Verification items for the finished model (mm, model axes). Face numbers are marked on the shaded views. Round coordinates to 2 decimals unless told otherwise and drop trailing zeros. Write each loop counter-clockwise with the first axis right and the second up, starting at its lowest first coordinate (ties: lowest second). Pieces come first, ordered by that corner, then holes. Notation, with made-up numbers: M 33,35.5 L 86,35.5 A14 ccw 86,60.5 Z; hole C 47.5,67.25 d10. An arc over 180 degrees is marked long. Answer in a Markdown table with one row per item. Add a question column.
1. Material ranges on probe 1 along Y at (x, z) = (0, 1.4) (3 decimals); probe 2 along X at (y, z) = (-0.75, 0.85); probe 3 along X at (y, z) = (1.25, 0.15), recorded low to high.
2. Sectioned sample at C-C on z = 1.05. Record the cut outline in (x, y) (3 decimals), plus the area to 3 significant figures.
3. Sectioned sample at B-B on y = 0. Record the cut outline in (x, z) (3 decimals), plus the area to 3 significant figures.
4. Draft check along Y on the marked faces 1, 2 and 3. Enter one of: pulls with the +Y half, pulls with the -Y half, needs draft (parallel to the pull), parting line crosses it, or undercut.
5. Sectioned sample at A-A on x = 0. Record the cut outline in (y, z) (3 decimals), plus the area to 4 significant figures.
```python
from build123d import *

# Parameters (mm, degrees)
F0_W     = 25.4
F0_H     = 12.7
F1_DEPTH = 2
F2_D     = 2.85
F3_D     = 3
F4_D     = 2.75


with BuildPart() as f1:
    # F0 (on Top) → F1 (new body)
    with BuildSketch(Plane.XY):
        Rectangle(F0_W, F0_H)
    extrude(amount=F1_DEPTH)

    # F2 (through all)
    with Locations(Plane(origin=(0, 0, 0), x_dir=(1, 0, 0), z_dir=(0, 0, -1))):
        with Locations((0, 0), (0, -6.35)):
            Hole(F2_D / 2)

    # F3 (through all)
    with Locations(Plane(origin=(0, 0, 0), x_dir=(1, 0, 0), z_dir=(0, 0, -1))):
        with Locations((8.2410294563, 0)):
            Hole(F3_D / 2)

    # F4 (through all)
    with Locations(Plane(origin=(0, 0, 0), x_dir=(1, 0, 0), z_dir=(0, 0, -1))):
        with Locations((-8.5610700771, 0)):
            Hole(F4_D / 2)


solid = f1.part
```
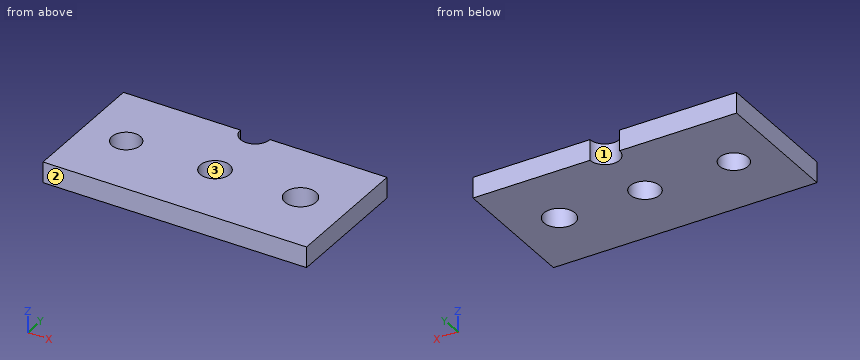
Geometry check:
| question | item | result |
|---|---|---|
| 1 | probe 1 | y = -6.35 to -1.425, 1.425 to 4.925 |
| 1 | probe 2 | x = -12.7 to -9.71, -7.41 to -1.21, 1.21 to 6.94, 9.54 to 12.7 |
| 1 | probe 3 | x = -12.7 to -9.13, -7.99 to -0.68, 0.68 to 7.41, 9.07 to 12.7 |
| 2 | outline | M -12.7,-6.35 L 12.7,-6.35 L 12.7,6.35 L 1.425,6.35 A1.425 cw -1.425,6.35 L -12.7,6.35 Z; hole C -8.561,0 d2.75; hole C 0,0 d2.85; hole C 8.241,0 d3 |
| 2 | area | 300 mm2 |
| 3 | outline | M -12.7,0 L -9.936,0 L -9.936,2 L -12.7,2 Z; M -7.186,0 L -1.425,0 L -1.425,2 L -7.186,2 Z; M 1.425,0 L 6.741,0 L 6.741,2 L 1.425,2 Z; M 9.741,0 L 12.7,0 L 12.7,2 L 9.741,2 Z |
| 3 | area | 33.6 mm2 |
| 4 | face 1 | pulls with the +Y half |
| 4 | face 2 | pulls with the -Y half |
| 4 | face 3 | undercut |
| 5 | outline | M -6.35,0 L -1.425,0 L -1.425,2 L -6.35,2 Z; M 1.425,0 L 4.925,0 L 4.925,2 L 1.425,2 Z |
| 5 | area | 16.85 mm2 |
